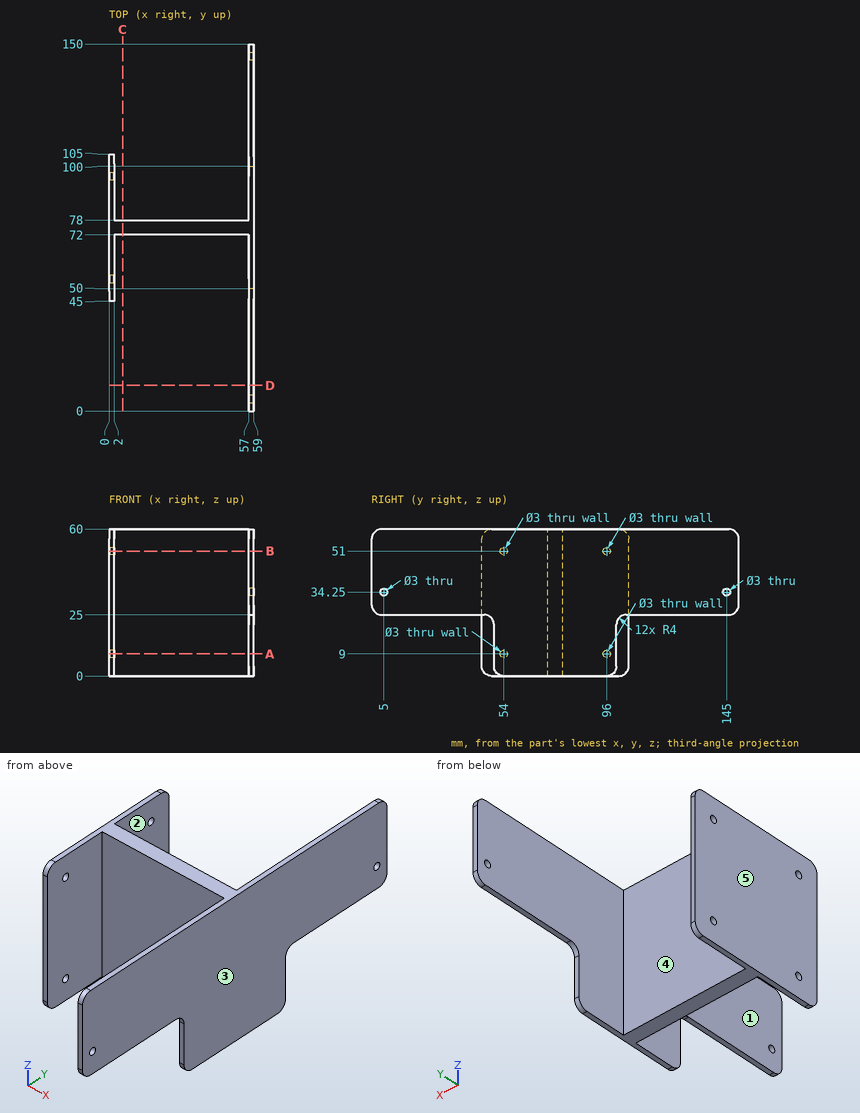
The figure shows three views and two pictorial views of one solid part (mm, origin at its lowest corner). Answer the questions. A direction names the side the tool comes from. Give positions to 0.01 mm unless a question says otherwise; leave off trailing zeros. Write each loop counter-clockwise with the first axis right and the second up, starting at its lowest first coordinate (ties: lowest second). Pieces come first, ordered by that corner, then holes. Notation, with made-up numbers: (11, 72.25) - (47, 72.25) arc R29 ccw to (47, 108.25) - close; hole circle Ø2 at (76.5, -28). An arc over 180 degrees is marked (long way). Use one line per item in the form item = value.
1. A cutting plane is placed at B-B (z = 51). Write down the section's boundary in (x, y).
Filled in:
outline = (0, 45) - (2, 45) - (2, 52.5) - (0, 52.5) - close; (0, 55.5) - (2, 55.5) - (2, 72) - (57, 72) - (57, 0) - (59, 0) - (59, 150) - (57, 150) - (57, 78) - (2, 78) - (2, 94.5) - (0, 94.5) - close; (0, 97.5) - (2, 97.5) - (2, 105) - (0, 105) - close
2. Consider L1, parallel to Z at x = 1.35, y = 54; L2, parallel to X at y = 96, z = 13; L3, parallel to Z at x = 58, y = 145. Determine where each line is inside the solid, lowest interval first.
Filled in:
L1 = 0 to 7.5, 10.5 to 49.5, 52.5 to 60
L2 = 0 to 2, 57 to 59
L3 = 25 to 32.75, 35.75 to 60
3. Each of these flat-tipped pins is pushed along its axis until it touches: pin 1 Ø1 at (x, z) = (1.5, 31) entering from -Y; pin 2 Ø2.5 at (y, z) = (96, 51) entering from -X; pin 3 Ø10 at (x, z) = (30.5, 19.5) entering from +Y; pin 4 Ø2.5 at (y, z) = (5, 34.25) entering from +X. Where does it stop, or does it pass through?
Filled in:
pin_1 = 45
pin_2 = 57
pin_3 = 78
pin_4 = through
4. Determine the mould class of the marked faces 3, 4 and 5 for opening direction X: released by +X, released by -X, zero draft, split by the parting line, or undercut.
Filled in:
face_3 = released by +X
face_4 = undercut
face_5 = released by -X
5. A cutting plane is placed at D-D (y = 10.5). Write down the section's boundary in (x, z).
Filled in:
outline = (57, 25) - (59, 25) - (59, 60) - (57, 60) - close
6. A cutting plane is placed at A-A (z = 9). Write down the section's boundary in (x, y).
Filled in:
outline = (0, 45) - (2, 45) - (2, 52.5) - (0, 52.5) - close; (0, 55.5) - (2, 55.5) - (2, 72) - (57, 72) - (57, 50) - (59, 50) - (59, 100) - (57, 100) - (57, 78) - (2, 78) - (2, 94.5) - (0, 94.5) - close; (0, 97.5) - (2, 97.5) - (2, 105) - (0, 105) - close
7. A cutting plane is placed at C-C (x = 5.5). Write down the section's boundary in (y, z), and give its area (3 significant figures).
Filled in:
outline = (72, 0) - (78, 0) - (78, 60) - (72, 60) - close
area = 360 mm^2
8. For the marked faces 1 and 2, determine the directions among +Z, -Z, +X, -X, +Y, -Y from which every point of the face is accessible in a straight line to the end or side of a thin tool.
Filled in:
face_1 = +Z, -Z, -Y
face_2 = +Z, -Z, +Y
